Here's how the part is built. I have some questions about the finished solid (model axes, mm). A direction names the side the tool comes from. Give positions to 0.01 mm unless a question says otherwise; leave off trailing zeros. Order: outer loops, then holes, each group sorted by start corner. A loop starts at its lowest first (then second) coordinate and runs counter-clockwise, first axis right, second up. Notation, with made-up numbers: M 34,-15 L 92,-15 A33 ccw 92,18 Z; hole C -35,3.5 d3. An arc over 180 degrees is marked long. Use one line per item in the form item = value.
from build123d import *

# Parameters (mm, degrees)
SKETCH1_R           = 2.4892
SKETCH1_R_2         = 2.5527
BOSS_EXTRUDE1_DEPTH = 3.175
FILLET1_R           = 4.7625


with BuildPart() as part:
    # Sketch1 → Boss-Extrude1 (new body)
    with BuildSketch(Plane.XY):
        Polygon((-33.401, 31.75), (-33.401, -29.21), (41.275, -29.21), (41.275, -7.62), (-17.145, -7.62), (-17.145, 31.75), align=None)
        with Locations((-25.4, -19.05)):
            Circle(SKETCH1_R, mode=Mode.SUBTRACT)
        with Locations((-7.9375, -19.05)):
            Circle(SKETCH1_R, mode=Mode.SUBTRACT)
        with Locations((-25.4, -6.35)):
            Circle(SKETCH1_R, mode=Mode.SUBTRACT)
        with Locations((9.525, -19.05)):
            Circle(SKETCH1_R_2, mode=Mode.SUBTRACT)
        with Locations((34.925, -19.05)):
            Circle(SKETCH1_R_2, mode=Mode.SUBTRACT)
        with Locations((-25.4, 6.35)):
            Circle(SKETCH1_R, mode=Mode.SUBTRACT)
        with Locations((-25.4, 19.05)):
            Circle(SKETCH1_R, mode=Mode.SUBTRACT)
        with Locations((-25.4, -19.05)):
            Circle(SKETCH1_R)
    extrude(amount=BOSS_EXTRUDE1_DEPTH)

    # Fillet1
    fillet1_edges = [part.edges().sort_by_distance(p)[0] for p in [
        (-33.401, 31.75, 1.5875),
        (-17.145, 31.75, 1.5875),
        (-17.145, -7.62, 1.5875),
        (41.275, -7.62, 1.5875),
        (41.275, -29.21, 1.5875),
        (-33.401, -29.21, 1.5875),
    ]]
    fillet(fillet1_edges, radius=FILLET1_R)


solid = part.part
Q1. I need wall thicknesses on L1, parallel to Y at x = -25.4, z = 1.5; L2, parallel to Y at x = -27, z = 0.6; L3, parallel to Y at x = 35, z = 0.55. Which ranges of each line are inside material? Lowest first, please.
Found:
L1 = -29.21 to -8.84, -3.86 to 3.86, 8.84 to 16.56, 21.54 to 31.75
L2 = -29.21 to -8.26, -4.44 to 4.44, 8.26 to 17.14, 20.96 to 31.75
L3 = -29.21 to -21.6, -16.5 to -7.62
Q2. On a 3-axis mill with a long thin cutter (end or side, diameter ignored), from which of +Z, -Z, +X, -X, +Y, -Y can I reach the whole of each face in a straight line? I mean faces 1 (the face through (41.275, -18, 2)), 2 (the face through (-17.145, 12, 2)). Say none if no direction works.
Found:
face_1 = +Z, -Z, +X, +Y, -Y
face_2 = +Z, -Z, +X, +Y
Q3. I want a section at C-C on x = -25.4. Write out the boundary of the cut face in (y, z) (3 decimals).
Found:
outline = M -29.21,0 L -8.839,0 L -8.839,3.175 L -29.21,3.175 Z; M -3.861,0 L 3.861,0 L 3.861,3.175 L -3.861,3.175 Z; M 8.839,0 L 16.561,0 L 16.561,3.175 L 8.839,3.175 Z; M 21.539,0 L 31.75,0 L 31.75,3.175 L 21.539,3.175 Z
Q4. Thinking about a two-plate mould opening in X: for faces 3 (the face through (-33.401, 2, 2)), 4 (the face through (-25, 31.75, 2)), 5 (the face through (-23.1, 18.1, 1.6)), 6 (the face through (-23.026, -5.602, 1.565)), which applies, +X half, -X half, draft (parallel to the pull), parting line (faces both ways), or undercut?
Found:
face_3 = -X half
face_4 = draft
face_5 = undercut
face_6 = undercut
Q5. I want a section at B-B on y = 19.05. Write out the boundary of the cut face in (x, z) (3 decimals).
Found:
outline = M -33.401,0 L -27.889,0 L -27.889,3.175 L -33.401,3.175 Z; M -22.911,0 L -17.145,0 L -17.145,3.175 L -22.911,3.175 Z
Q6. I want a section at A-A on y = -19.05. Write out the boundary of the cut face in (x, z) (3 decimals).
Found:
outline = M -33.401,0 L -10.427,0 L -10.427,3.175 L -33.401,3.175 Z; M -5.448,0 L 6.972,0 L 6.972,3.175 L -5.448,3.175 Z; M 12.078,0 L 32.372,0 L 32.372,3.175 L 12.078,3.175 Z; M 37.478,0 L 41.275,0 L 41.275,3.175 L 37.478,3.175 Z
Q7. I want a section at D-D on z = 0.85. State how many separate pieces and enclosed holes the cut face has, then the cut area to 3 significant figures.
Found:
separate_pieces = 1
enclosed_holes = 6
area = 2,110 mm²
